```python
from build123d import *

# Parameters (mm, degrees)
EXTRUDE_1_DEPTH = 10
EXTRUDE_2_DEPTH = 13


with BuildPart() as part:
    # Эскиз1 → Повернуть1 (revolve)
    with BuildSketch(Plane.XY, mode=Mode.PRIVATE) as revolve_1_sk:
        Polygon((0, 0), (-49.8, 0), (-49.8, 2), (-50, 2), (-50, 8), (-20, 29), (-8, 29), (-8, 39), (-8, 187), (-6, 189), (0, 189), align=None)
    revolve(revolve_1_sk.sketch.rotate(Axis((0, 0, 0), (0, 1, 0)), 180), axis=Axis((0, 0, 0), (0, 1, 0)))  # turned: the seam where the file's is

    # Эскиз2 → Бобышка-Вытянуть1 (add)
    with BuildSketch(Plane(origin=(0, 29, 0), x_dir=(1, 0, 0), z_dir=(0, 1, 0))):
        Polygon((0, 13.856406461), (-12, 6.92820323), (-12, -6.92820323), (0, -13.856406461), (12, -6.92820323), (12, 6.92820323), align=None)
    extrude(amount=EXTRUDE_1_DEPTH)

    # Эскиз3 → Бобышка-Вытянуть2 (add)
    with BuildSketch(Plane(origin=(0, 113, 0), x_dir=(1, 0, 0), z_dir=(0, 1, 0))):
        Polygon((12, 6.92820323), (0, 13.856406461), (-12, 6.92820323), (-12, -6.92820323), (0, -13.856406461), (12, -6.92820323), align=None)
    extrude(amount=EXTRUDE_2_DEPTH)

    # Эскиз4 → Вырез-Повернуть2 (revolve, cut)
    with BuildSketch(Plane.XY, mode=Mode.PRIVATE) as cut_revolve_2_sk:
        Polygon((-23.258330249, 126), (-12, 126), (-23.258330249, 119.5), align=None)
        Polygon((-23.258330249, 113), (-23.258330249, 119.5), (-12, 113), align=None)
        Polygon((-20.660254038, 39), (-20.660254038, 34), (-12, 39), align=None)
        Polygon((-20.660254038, 34), (-20.660254038, 29), (-12, 29), align=None)
    revolve(cut_revolve_2_sk.sketch.rotate(Axis((0, 189, 0), (0, -1, 0)), 180), axis=Axis((0, 189, 0), (0, -1, 0)), mode=Mode.SUBTRACT)  # turned: the seam where the file's is


solid = part.part
```
For this review, take the finished solid that the model builds, in its own axes (mm). A direction names the side the tool comes from. Round coordinates to 2 decimals unless told otherwise and drop trailing zeros. Write each loop counter-clockwise with the first axis right and the second up, starting at its lowest first coordinate (ties: lowest second). Pieces come first, ordered by that corner, then holes. Notation, with made-up numbers: (-10, 60) -> (-2, 60) arc R11 cw to (-2, 64) -> close; hole circle Ø11 at (40, -20.75). An arc over 180 degrees is marked (long way). One line per question, with ' | ' between items. Start each with the question number.
1) For pin 1 Ø8 at (x, y) = (0, 62) entering from -Z; pin 2 Ø4 at (y, z) = (120, 0) entering from +X; pin 3 Ø4 at (x, z) = (-34.5, 2) entering from +Y, all flat-tipped, find the tip position at first contact; note any pin that passes through.
2) Wall thickness on line 1 along X through (y, z) = (122.5, 6.5); line 2 along Y through (x, z) = (-16.5, -6); line 3 along X through (y, z) = (154, -5) (3 decimals): over which ranges is each line inside the solid? List them lowest first.
3) Machinability: for faces 1 (the flat face through (-6.084, 33.93, 10.344)), 2 (the cylindrical face through (22.98, 1.01, 44.18)), 3 (the conical face through (-10.791, 38.744, -6.195)), which of the approach directions +Z, -Z, +X, -X, +Y, -Y give a long, thin tool a straight path to every point of the face, cutting with its end or side? Answer none if there is none.
4) Add section B-B (y = 25). Write out the cut boundary in (x, z), and give its area (3 significant figures).
5) Add section A-A (y = 98). Write out the cut boundary in (x, z).
Reported:
1) pin 1: stops at z = -8 | pin 2: stops at x = 12 | pin 3: stops at y = 20.21
2) line 1: x = -12 to 12 | line 2: y = 0 to 29 | line 3: x = -6.245 to 6.245
3) face 1: +Z, -X, +Y | face 2: -Y | face 3: -Z, -X
4) outline: circle Ø51.43 at (0, 0) | area: 2,080 mm²
5) outline: circle Ø16 at (0, 0)
